from build123d import *

# Parameters (mm, degrees)
SKETCH_1_R             = 14
EXTRUDE_1_DEPTH        = 5
SKETCH_2_W             = 2
SKETCH_2_H             = 25
EXTRUDE_2_DEPTH        = 1
CUT_EXTRUDE_2_REACH    = 7
HOLE_WIZARD_M3_1_D     = 2.5
HOLE_WIZARD_M3_1_DEPTH = 8.5
HOLE_WIZARD_M3_1_TIP   = 0.751075774
SKETCH_9_R             = 14
EXTRUDE_3_DEPTH        = 1
HOLE_WIZARD_M3_3_D     = 2.5
HOLE_WIZARD_M3_3_DEPTH = 8.5
HOLE_WIZARD_M3_3_TIP   = 0.751075774
CUT_EXTRUDE_3_REACH    = 7
SKETCH_12_R            = 1.6
SKETCH_13_R            = 3
CUT_EXTRUDE_4_DEPTH    = 3


with BuildPart() as part:
    # 草图1 → 凸台-拉伸1 (new body)
    with BuildSketch(Plane.XY):
        with BuildLine():
            Line((-85, 25), (-85, 50))
            Line((-85, 50), (-76, 50))
            Line((-76, 50), (-35.333333333, 19.5))
            ThreePointArc((-35.333333333, 19.5), (-32.495610994, 18.013167019), (-29.333333333, 17.5))
            Line((-29.333333333, 17.5), (29.333333333, 17.5))
            ThreePointArc((29.333333333, 17.5), (32.495610994, 18.013167019), (35.333333333, 19.5))
            Line((35.333333333, 19.5), (76, 50))
            Line((76, 50), (85, 50))
            Line((85, 50), (85, 25))
            Line((85, 25), (76, 25))
            Line((76, 25), (49.00243962, -8.746950476))
            ThreePointArc((49.00243962, -8.746950476), (45.52563883, -11.513032363), (41.193751525, -12.5))
            Line((41.193751525, -12.5), (31, -12.5))
            Line((31, -12.5), (26, -17.5))
            Line((26, -17.5), (-26, -17.5))
            Line((-26, -17.5), (-31, -12.5))
            Line((-31, -12.5), (-41.193751525, -12.5))
            ThreePointArc((-41.193751525, -12.5), (-45.52563883, -11.513032363), (-49.00243962, -8.746950476))
            Line((-49.00243962, -8.746950476), (-76, 25))
            Line((-76, 25), (-85, 25))
        make_face()
        Circle(SKETCH_1_R, mode=Mode.SUBTRACT)
    extrude(amount=EXTRUDE_1_DEPTH)

    # 草图2 → 凸台-拉伸2 (add)
    with BuildSketch(Plane.XY.offset(5)):
        with Locations((-77, 37.5)):
            Rectangle(SKETCH_2_W, SKETCH_2_H)
        with Locations((77, 37.5)):
            Rectangle(SKETCH_2_W, SKETCH_2_H)
    extrude(amount=EXTRUDE_2_DEPTH)

    # 草图3 → 切除-拉伸2 (cut, up to next)
    with BuildSketch(Plane.XY.offset(5), mode=Mode.PRIVATE) as cut_extrude_2_sk1:
        with BuildLine():
            Line((-71.624088, 28.017247632), (-53.714483662, 8.288938763))
            ThreePointArc((-53.714483662, 8.288938763), (-50.037049276, 6.649771189), (-46.343650352, 8.252643109))
            Line((-46.343650352, 8.252643109), (-44.561564605, 10.177266985))
            ThreePointArc((-44.561564605, 10.177266985), (-43.247059214, 13.982850984), (-45.163793368, 17.523546422))
            Line((-45.163793368, 17.523546422), (-66.209204362, 33.865234658))
            ThreePointArc((-66.209204362, 33.865234658), (-71.597466294, 33.423519047), (-71.624088, 28.017247632))
        make_face()
    cut_extrude_2_tool1 = extrude(cut_extrude_2_sk1.sketch, amount=-CUT_EXTRUDE_2_REACH, mode=Mode.PRIVATE) & part.part
    add(cut_extrude_2_tool1.solids().sort_by_distance((-57.416432, 20.292736, 5))[0], mode=Mode.SUBTRACT)
    # 草图3 → 切除-拉伸2 (cut, up to next)
    with BuildSketch(Plane.XY.offset(5), mode=Mode.PRIVATE) as cut_extrude_2_sk2:
        with BuildLine():
            Line((44.878567193, 3.211549518), (46.335374238, 1.638221397))
            ThreePointArc((46.335374238, 1.638221397), (45.673933781, -0.192361307), (44.563707744, -1.791090382))
            ThreePointArc((44.563707744, -1.791090382), (33.507457779, -1.845533864), (34.410800923, 9.173885293))
            ThreePointArc((34.410800923, 9.173885293), (36.090068224, 10.158058978), (37.966040159, 10.676967267))
            Line((37.966040159, 10.676967267), (44.878567193, 3.211549518))
        make_face()
    cut_extrude_2_tool2 = extrude(cut_extrude_2_sk2.sketch, amount=-CUT_EXTRUDE_2_REACH, mode=Mode.PRIVATE) & part.part
    add(cut_extrude_2_tool2.solids().sort_by_distance((38.242863, 2.539166, 5))[0], mode=Mode.SUBTRACT)
    # 草图3 → 切除-拉伸2 (cut, up to next)
    with BuildSketch(Plane.XY.offset(5), mode=Mode.PRIVATE) as cut_extrude_2_sk3:
        with BuildLine():
            Line((-44.878567193, 3.211549518), (-46.335374238, 1.638221397))
            ThreePointArc((-46.335374238, 1.638221397), (-45.673933781, -0.192361307), (-44.563707744, -1.791090382))
            ThreePointArc((-44.563707744, -1.791090382), (-33.507457779, -1.845533864), (-34.410800923, 9.173885293))
            ThreePointArc((-34.410800923, 9.173885293), (-36.090068224, 10.158058978), (-37.966040159, 10.676967267))
            Line((-37.966040159, 10.676967267), (-44.878567193, 3.211549518))
        make_face()
    cut_extrude_2_tool3 = extrude(cut_extrude_2_sk3.sketch, amount=-CUT_EXTRUDE_2_REACH, mode=Mode.PRIVATE) & part.part
    add(cut_extrude_2_tool3.solids().sort_by_distance((-38.242863, 2.539166, 5))[0], mode=Mode.SUBTRACT)
    # 草图3 → 切除-拉伸2 (cut, up to next)
    with BuildSketch(Plane.XY.offset(5), mode=Mode.PRIVATE) as cut_extrude_2_sk4:
        with BuildLine():
            Line((46.343650352, 8.252643109), (44.561564605, 10.177266985))
            ThreePointArc((44.561564605, 10.177266985), (43.247059214, 13.982850984), (45.163793368, 17.523546422))
            Line((45.163793368, 17.523546422), (66.209204362, 33.865234658))
            ThreePointArc((66.209204362, 33.865234658), (71.597466294, 33.423519047), (71.624088, 28.017247632))
            Line((71.624088, 28.017247632), (53.714483662, 8.288938763))
            ThreePointArc((53.714483662, 8.288938763), (50.037049276, 6.649771189), (46.343650352, 8.252643109))
        make_face()
    cut_extrude_2_tool4 = extrude(cut_extrude_2_sk4.sketch, amount=-CUT_EXTRUDE_2_REACH, mode=Mode.PRIVATE) & part.part
    add(cut_extrude_2_tool4.solids().sort_by_distance((57.416432, 20.292736, 5))[0], mode=Mode.SUBTRACT)

    # M3 螺纹孔1
    with Locations(Plane(origin=(-42, 10, 5), x_dir=(1, 0, 0), z_dir=(0, 0, 1))):
        with Locations((0, 0), (0, -20), (84, 0), (84, -20)):
            Hole(HOLE_WIZARD_M3_1_D / 2, depth=HOLE_WIZARD_M3_1_DEPTH)
            with Locations((0, 0, -(HOLE_WIZARD_M3_1_DEPTH + HOLE_WIZARD_M3_1_TIP / 2))):  # 118° drill point
                Cone(0, HOLE_WIZARD_M3_1_D / 2, HOLE_WIZARD_M3_1_TIP, mode=Mode.SUBTRACT)

    # 草图9 → 凸台-拉伸3 (add)
    with BuildSketch(Plane.XY.offset(5)):
        with BuildLine():
            Line((-31, -12.5), (-31, 17.639867028))
            ThreePointArc((-31, 17.639867028), (-30.169595936, 17.535028105), (-29.333333333, 17.5))
            Line((-29.333333333, 17.5), (29.333333333, 17.5))
            ThreePointArc((29.333333333, 17.5), (30.169595936, 17.535028105), (31, 17.639867028))
            Line((31, 17.639867028), (31, -12.5))
            Line((31, -12.5), (26, -17.5))
            Line((26, -17.5), (-26, -17.5))
            Line((-26, -17.5), (-31, -12.5))
        make_face()
        Circle(SKETCH_9_R, mode=Mode.SUBTRACT)
    extrude(amount=EXTRUDE_3_DEPTH)

    # M3 螺纹孔3
    with Locations(Plane(origin=(-23, 7.5, 6), x_dir=(1, 0, 0), z_dir=(0, 0, 1))):
        with Locations((0, 0), (0, -15), (46, -15), (46, 0)):
            Hole(HOLE_WIZARD_M3_3_D / 2, depth=HOLE_WIZARD_M3_3_DEPTH)
            with Locations((0, 0, -(HOLE_WIZARD_M3_3_DEPTH + HOLE_WIZARD_M3_3_TIP / 2))):  # 118° drill point
                Cone(0, HOLE_WIZARD_M3_3_D / 2, HOLE_WIZARD_M3_3_TIP, mode=Mode.SUBTRACT)

    # 草图12 → 切除-拉伸3 (cut, up to next)
    with BuildSketch(Plane.XY.offset(5), mode=Mode.PRIVATE) as cut_extrude_3_sk1:
        with Locations((-81.5, 37.5)):
            Circle(SKETCH_12_R)
    cut_extrude_3_tool1 = extrude(cut_extrude_3_sk1.sketch, amount=-CUT_EXTRUDE_3_REACH, mode=Mode.PRIVATE) & part.part
    add(cut_extrude_3_tool1.solids().sort_by_distance((-81.5, 37.5, 5))[0], mode=Mode.SUBTRACT)
    # 草图12 → 切除-拉伸3 (cut, up to next)
    with BuildSketch(Plane.XY.offset(5), mode=Mode.PRIVATE) as cut_extrude_3_sk2:
        with Locations((-81.5, 29)):
            Circle(SKETCH_12_R)
    cut_extrude_3_tool2 = extrude(cut_extrude_3_sk2.sketch, amount=-CUT_EXTRUDE_3_REACH, mode=Mode.PRIVATE) & part.part
    add(cut_extrude_3_tool2.solids().sort_by_distance((-81.5, 29, 5))[0], mode=Mode.SUBTRACT)
    # 草图12 → 切除-拉伸3 (cut, up to next)
    with BuildSketch(Plane.XY.offset(5), mode=Mode.PRIVATE) as cut_extrude_3_sk3:
        with Locations((-81.5, 46)):
            Circle(SKETCH_12_R)
    cut_extrude_3_tool3 = extrude(cut_extrude_3_sk3.sketch, amount=-CUT_EXTRUDE_3_REACH, mode=Mode.PRIVATE) & part.part
    add(cut_extrude_3_tool3.solids().sort_by_distance((-81.5, 46, 5))[0], mode=Mode.SUBTRACT)
    # 草图12 → 切除-拉伸3 (cut, up to next)
    with BuildSketch(Plane.XY.offset(5), mode=Mode.PRIVATE) as cut_extrude_3_sk4:
        with Locations((81.5, 46)):
            Circle(SKETCH_12_R)
    cut_extrude_3_tool4 = extrude(cut_extrude_3_sk4.sketch, amount=-CUT_EXTRUDE_3_REACH, mode=Mode.PRIVATE) & part.part
    add(cut_extrude_3_tool4.solids().sort_by_distance((81.5, 46, 5))[0], mode=Mode.SUBTRACT)
    # 草图12 → 切除-拉伸3 (cut, up to next)
    with BuildSketch(Plane.XY.offset(5), mode=Mode.PRIVATE) as cut_extrude_3_sk5:
        with Locations((81.5, 29)):
            Circle(SKETCH_12_R)
    cut_extrude_3_tool5 = extrude(cut_extrude_3_sk5.sketch, amount=-CUT_EXTRUDE_3_REACH, mode=Mode.PRIVATE) & part.part
    add(cut_extrude_3_tool5.solids().sort_by_distance((81.5, 29, 5))[0], mode=Mode.SUBTRACT)
    # 草图12 → 切除-拉伸3 (cut, up to next)
    with BuildSketch(Plane.XY.offset(5), mode=Mode.PRIVATE) as cut_extrude_3_sk6:
        with Locations((81.5, 37.5)):
            Circle(SKETCH_12_R)
    cut_extrude_3_tool6 = extrude(cut_extrude_3_sk6.sketch, amount=-CUT_EXTRUDE_3_REACH, mode=Mode.PRIVATE) & part.part
    add(cut_extrude_3_tool6.solids().sort_by_distance((81.5, 37.5, 5))[0], mode=Mode.SUBTRACT)

    # 草图13 → 切除-拉伸4 (cut)
    with BuildSketch(Plane(origin=(0, 0, 0), x_dir=(-1, 0, 0), z_dir=(0, 0, -1))):
        with Locations((-81.5, 37.5)):
            Circle(SKETCH_13_R)
        with Locations((-81.5, 46)):
            Circle(SKETCH_13_R)
        with Locations((-81.5, 29)):
            Circle(SKETCH_13_R)
        with Locations((81.5, 29)):
            Circle(SKETCH_13_R)
        with Locations((81.5, 37.5)):
            Circle(SKETCH_13_R)
        with Locations((81.5, 46)):
            Circle(SKETCH_13_R)
    extrude(amount=-CUT_EXTRUDE_4_DEPTH, mode=Mode.SUBTRACT)


solid = part.part
Here's how the part is built. I have some questions about the finished solid (model axes, mm). A direction names the side the tool comes from. Round coordinates to 2 decimals unless told otherwise and drop trailing zeros. Write each loop counter-clockwise with the first axis right and the second up, starting at its lowest first coordinate (ties: lowest second). Pieces come first, ordered by that corner, then holes.
1. Will these pins go through, and if not, where does the flat tip stop? pin 1 Ø3.5 at (x, y) = (-80.5, 31.5) entering from +Z; pin 2 Ø3 at (x, y) = (81.5, 45.5) entering from -Z.
2. If we mould it in two halves opening along X, with no side actions, what happens to faces 6 (the cylindrical face through (84.5, 29.1, 1.5)), 7 (the flat face through (-81, 25, 3)), 8 (the flat face through (-28.5, -15, 3))? For each: released by +X, released by -X, zero draft, split by the parting line, or undercut.
3. For faces 1 (the flat face through (62.8, 18.3, 2.5)), 2 (the flat face through (-48, 21, 5)), 3 (the flat face through (36, -12.5, 2)), 4 (the flat face through (84, 38, 5)), 5 (the cylindrical face through (-79.29, 39.53, 1.48)), which set-ups out of +Z, -Z, +X, -X, +Y, -Y let a thin tool reach every point of the face, with its end or its side?
4. Suppose I cut it at B-B (y = 0). List the corners of the cut face in (x, z) for me.
5. I need wall thicknesses on L1, parallel to Y at x = -81.5, z = 1.8; L2, parallel to X at y = 31, z = 0.6; L3, parallel to X at y = 39.5, z = 1.85. Which ranges of each line are inside material? Lowest first, please.
6. Suppose I cut it at D-D (x = 50.5). List the corners of the cut face in (y, z) for me (3 decimals).
7. Suppose I cut it at C-C (x = -64.5). List the corners of the cut face in (y, z) for me (3 decimals), and give its area (3 significant figures).
8. Suppose I cut it at A-A (x = 81.5). List the corners of the cut face in (y, z) for me.
Answer sheet:
1. pin 1: stops at z = 5
1. pin 2: stops at z = 3
2. face 6: undercut
2. face 7: zero draft
2. face 8: released by -X
3. face 1: +Z, -Z
3. face 2: +Z, +Y, -Y
3. face 3: +Z, -Z, +X, -Y
3. face 4: +Z, +X, +Y, -Y
3. face 5: -Z
4. outline: (-56, 0) - (-45.77, 0) - (-45.77, 5) - (-56, 5) - close; (-32.25, 0) - (-14, 0) - (-14, 6) - (-31, 6) - (-31, 5) - (-32.25, 5) - close; (14, 0) - (32.25, 0) - (32.25, 5) - (31, 5) - (31, 6) - (14, 6) - close; (45.77, 0) - (56, 0) - (56, 5) - (45.77, 5) - close
5. L1: y = 25 to 26, 32 to 34.5, 40.5 to 43, 49 to 50
5. L2: x = -85 to -83.74, -79.26 to -72.65, -62.52 to -50.67, 50.67 to 62.52, 72.65 to 79.26, 83.74 to 85
5. L3: x = -85 to -83.74, -79.26 to -62, 62 to 79.26, 83.74 to 85
6. outline: (-6.875, 0) - (6.674, 0) - (6.674, 5) - (-6.875, 5) - close; (21.667, 0) - (30.875, 0) - (30.875, 5) - (21.667, 5) - close
7. outline: (10.625, 0) - (20.17, 0) - (20.17, 5) - (10.625, 5) - close; (32.538, 0) - (41.375, 0) - (41.375, 5) - (32.538, 5) - close
7. area: 91.9 mm2
8. outline: (25, 0) - (26, 0) - (26, 3) - (27.4, 3) - (27.4, 5) - (25, 5) - close; (30.6, 3) - (32, 3) - (32, 0) - (34.5, 0) - (34.5, 3) - (35.9, 3) - (35.9, 5) - (30.6, 5) - close; (39.1, 3) - (40.5, 3) - (40.5, 0) - (43, 0) - (43, 3) - (44.4, 3) - (44.4, 5) - (39.1, 5) - close; (47.6, 3) - (49, 3) - (49, 0) - (50, 0) - (50, 5) - (47.6, 5) - close
